Geometry: final body of the model. Coordinates: model frame, mm. Round coordinates to 2 decimals unless told otherwise and drop trailing zeros. Loops run counter-clockwise (first coordinate to the right, second up) from the corner with the lowest first, then second, coordinate; pieces in that order, holes last. Notation, with made-up numbers: (-5, 58) -> (27, 58) arc R12 ccw to (27, 63) -> close; hole circle Ø4 at (71, 38.5). An arc over 180 degrees is marked (long way). Answer in a Markdown table with one row per item.
```python
from build123d import *

# Parameters (mm, degrees)
SKETCH1_W        = 50.8
SKETCH1_H        = 25.4
BLOCK_DEPTH      = 19.05
SKETCH2_R        = 12.7
SHAFTHOLE_DEPTH  = 41.659838908
CLAMPING_HOLES_D = 6.35


with BuildPart() as part:
    # Sketch1 → Block (new body)
    with BuildSketch(Plane(origin=(0, 0, 0), x_dir=(1, 0, 0), z_dir=(0, 1, 0))):
        Rectangle(SKETCH1_W, SKETCH1_H)
    extrude(amount=BLOCK_DEPTH)

    # Sketch2 → ShaftHole (cut, through all)
    with BuildSketch(Plane.XY.offset(12.7)):
        with Locations((0, -0.127)):
            Circle(SKETCH2_R)
    extrude(amount=-SHAFTHOLE_DEPTH, mode=Mode.SUBTRACT)

    # Clamping Holes (through all)
    with Locations(Plane(origin=(0, 19.05, 0), x_dir=(1, 0, 0), z_dir=(0, 1, 0))):
        with Locations((-19.05, 0), (19.05, 0)):
            Hole(CLAMPING_HOLES_D / 2)


solid = part.part
```
Item 1: Cut plane A-A (z = 0). Output: boundary loops of the cut face in (x, y) (3 decimals).
Answer:
| item | result |
|---|---|
| outline | (-25.4, 0) -> (-22.225, 0) -> (-22.225, 19.05) -> (-25.4, 19.05) -> close; (-15.875, 0) -> (-12.699, 0) arc R12.7 cw to (12.699, 0) -> (15.875, 0) -> (15.875, 19.05) -> (-15.875, 19.05) -> close; (22.225, 0) -> (25.4, 0) -> (25.4, 19.05) -> (22.225, 19.05) -> close |
Item 2: Cut plane C-C (y = 8). Output: boundary loops of the cut face in (x, z) (3 decimals).
Answer:
| item | result |
|---|---|
| outline | (-25.4, -12.7) -> (-9.759, -12.7) -> (-9.759, 12.7) -> (-25.4, 12.7) -> close; (9.759, -12.7) -> (25.4, -12.7) -> (25.4, 12.7) -> (9.759, 12.7) -> close; hole circle Ø6.35 at (-19.05, 0); hole circle Ø6.35 at (19.05, 0) |
Item 3: Draft query along X for faces 1 (the face through (25.4, 9, 0)), 2 (the face through (16.02, 9.39, -0.95)), 3 (the face through (-15.88, 9.39, -0.14)), 4 (the face through (-21, 0, -3)). Return one class per face: pulls with the +X half, pulls with the -X half, needs draft (parallel to the pull), parting line crosses it, or undercut.
Answer:
| item | result |
|---|---|
| face 1 | pulls with the +X half |
| face 2 | undercut |
| face 3 | undercut |
| face 4 | needs draft |
Item 4: Line query: probe 1 along Z at (x, y) = (19.05, 12) (3 decimals); probe 2 along Z at (x, y) = (-17, 7); probe 3 along X at (y, z) = (17, 0.75). Output: solid intervals per line, ascending. Write a range as [from, to].
Answer:
| item | result |
|---|---|
| probe 1 | z = [-12.7, -3.175], [3.175, 12.7] |
| probe 2 | z = [-12.7, -2.42], [2.42, 12.7] |
| probe 3 | x = [-25.4, -22.14], [-15.96, 15.96], [22.14, 25.4] |
Item 5: Cut plane D-D (y = 15). Output: boundary loops of the cut face in (x, z) (3 decimals).
Answer:
| item | result |
|---|---|
| outline | (-25.4, -12.7) -> (25.4, -12.7) -> (25.4, 12.7) -> (-25.4, 12.7) -> close; hole circle Ø6.35 at (-19.05, 0); hole circle Ø6.35 at (19.05, 0) |
Item 6: Pin query (flat end, axial travel): pin 1 Ø5.5 at (x, z) = (-19.05, 0) entering from +Y. Return the tip coordinate at first contact, or that it passes through.
Answer:
| item | result |
|---|---|
| pin 1 | passes through |
Item 7: Cut plane B-B (x = -19.05). Output: boundary loops of the cut face in (y, z) (3 decimals).
Answer:
| item | result |
|---|---|
| outline | (0, -12.7) -> (19.05, -12.7) -> (19.05, -3.175) -> (0, -3.175) -> close; (0, 3.175) -> (19.05, 3.175) -> (19.05, 12.7) -> (0, 12.7) -> close |
